Work out the finished part from the listing and answer in its coordinate system (mm). Face numbers are marked on the shaded views. A direction names the side the tool comes from. Round coordinates to 2 decimals unless told otherwise and drop trailing zeros. Order: outer loops, then holes, each group sorted by start corner. A loop starts at its lowest first (then second) coordinate and runs counter-clockwise, first axis right, second up. Notation, with made-up numbers: (60, 88.25) - (97, 88.25) arc R32 ccw to (97, 121.25) - close; hole circle Ø7 at (11.5, -11.75). An arc over 180 degrees is marked (long way). Put each result on its own line as item: value.
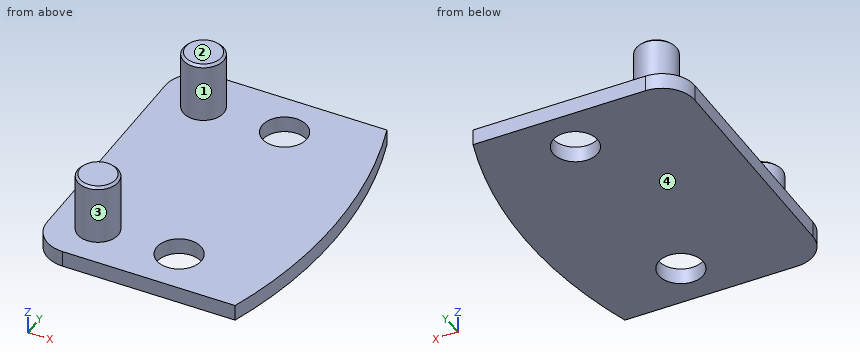
Autodesk Inventor part; units mm, degrees
ref_plane "YZ Plane" through (0, 0, 0) normal (1, 0, 0) x (0, 1, 0)
ref_plane "XZ Plane" through (0, 0, 0) normal (0, 1, 0) x (-1, 0, 0)
ref_plane "XY Plane" through (0, 0, 0) normal (0, 0, 1) x (1, 0, 0)
sketch "Esquisse1" plane through (0, 0, 0) normal (0, 0, 1) x (1, 0, 0)
  line L0 (0, 0) -> (-29, 0)
  line L1 (-29, 0) -> (-29, 36)
  line L2 (-29, 36) -> (0, 36)
  line L3 (-24.5656, 33) -> (-19.5656, 33)
  line L4 (-19.5656, 33) -> (-19.5656, 28)
  line L5 (-19.5656, 28) -> (-24.5656, 28)
  line L6 (-24.5656, 28) -> (-24.5656, 33)
  line L7 (-14.5656, 33) -> (-9.5656, 33)
  line L8 (-9.5656, 33) -> (-9.5656, 28)
  line L9 (-9.5656, 28) -> (-14.5656, 28)
  line L10 (-14.5656, 28) -> (-14.5656, 33)
  line L11 (-24.5656, 8) -> (-19.5656, 8)
  line L12 (-19.5656, 8) -> (-19.5656, 3)
  line L13 (-19.5656, 3) -> (-24.5656, 3)
  line L14 (-24.5656, 3) -> (-24.5656, 8)
  line L15 (-14.5656, 8) -> (-9.5656, 8)
  line L16 (-9.5656, 8) -> (-9.5656, 3)
  line L17 (-9.5656, 3) -> (-14.5656, 3)
  line L18 (-14.5656, 3) -> (-14.5656, 8)
  arc A0 (0, 0) -> (0, 36) centre (-54.0833, 18) ccw
  line L19 (-9.3156, 33.25) -> (-14.8156, 33.25)
  line L20 (-14.8156, 33.25) -> (-14.8156, 27.75)
  line L21 (-14.8156, 27.75) -> (-9.3156, 27.75)
  line L22 (-9.3156, 27.75) -> (-9.3156, 33.25)
  line L23 (-9.3156, 8.25) -> (-14.8156, 8.25)
  line L24 (-14.8156, 8.25) -> (-14.8156, 2.75)
  line L25 (-14.8156, 2.75) -> (-9.3156, 2.75)
  line L26 (-9.3156, 2.75) -> (-9.3156, 8.25)
  dimension "d0" = 36
  dimension "d1" = 29
  dimension "d2" = 5
  dimension "d3" = 5
  dimension "d4" = 5
  dimension "d5" = 5
  dimension "d6" = 20
  dimension "d7" = 5
  dimension "d8" = 3
  dimension "d9" = 57
  dimension "d21" = 5.5
  dimension "d22" = 5.5
extrude "Extrusion1" add sketch "Esquisse1" along normal blind 2 contours L0 L1 L2 A0 | L22 L21 L20 L19 | L26 L25 L24 L23
extrude "Extrusion3" add sketch "Esquisse1" along normal blind 9.5 contours L3 L4 L5 L6 | L11 L12 L13 L14
fillet "Congé1" radius 4 2 edges at (-29, 0, 1) (-29, 36, 1)
sketch "Esquisse2" plane through (0, 0, 2) normal (0, 0, 1) x (1, 0, 0)
  line L0 (-9.5656, 8) -> (-9.5656, 3)
  line L1 (-9.5656, 3) -> (-14.5656, 3)
  line L2 (-14.5656, 3) -> (-14.5656, 8)
  line L3 (-14.5656, 8) -> (-9.5656, 8)
  line L4 (-19.5656, 8) -> (-19.5656, 3)
  line L5 (-19.5656, 3) -> (-24.5656, 3)
  line L6 (-24.5656, 3) -> (-24.5656, 8)
  line L7 (-24.5656, 8) -> (-19.5656, 8)
  line L8 (-9.5656, 33) -> (-9.5656, 28)
  line L9 (-9.5656, 28) -> (-14.5656, 28)
  line L10 (-14.5656, 28) -> (-14.5656, 33)
  line L11 (-14.5656, 33) -> (-9.5656, 33)
  line L12 (-19.5656, 33) -> (-19.5656, 28)
  line L13 (-19.5656, 28) -> (-24.5656, 28)
  line L14 (-24.5656, 28) -> (-24.5656, 33)
  line L15 (-24.5656, 33) -> (-19.5656, 33)
  arc A0 (-25, 36) -> (-29, 32) centre (-25, 32) ccw
  line L16 (-29, 32) -> (-29, 4)
  arc A1 (-29, 4) -> (-25, 0) centre (-25, 4) ccw
  line L17 (-25, 0) -> (0, 0)
  arc A2 (0, 0) -> (0, 36) centre (-54.0833, 18) ccw
  line L18 (0, 36) -> (-25, 36)
  circle A3 centre (-12.0656, 30.5) radius 2.5
  circle A4 centre (-12.0656, 5.5) radius 2.5
extrude "Extrusion4" add sketch "Esquisse2" against normal up to surface (2 mm away) contours L0 A4 L3 | L0 L1 A4 | A4 L2 L3 | L1 L2 A4 | L8 A3 L11 | L8 L9 A3 | A3 L10 L11 | L9 L10 A3
sketch "Esquisse3" plane through (0, 0, 9.5) normal (0, 0, 1) x (1, 0, 0)
  circle A0 centre (-12.0656, 5.5) radius 2.5
  line L0 (-19.5656, 8) -> (-19.5656, 3)
  line L1 (-19.5656, 3) -> (-24.5656, 3)
  line L2 (-24.5656, 3) -> (-24.5656, 8)
  line L3 (-24.5656, 8) -> (-19.5656, 8)
  circle A1 centre (-12.0656, 30.5) radius 2.5
  line L4 (-19.5656, 33) -> (-19.5656, 28)
  line L5 (-19.5656, 28) -> (-24.5656, 28)
  line L6 (-24.5656, 28) -> (-24.5656, 33)
  line L7 (-24.5656, 33) -> (-19.5656, 33)
  arc A2 (-25, 36) -> (-29, 32) centre (-25, 32) ccw
  line L8 (-29, 32) -> (-29, 4)
  arc A3 (-29, 4) -> (-25, 0) centre (-25, 4) ccw
  line L9 (-25, 0) -> (0, 0)
  arc A4 (0, 0) -> (0, 36) centre (-54.0833, 18) ccw
  line L10 (0, 36) -> (-25, 36)
  circle A5 centre (-22.0656, 30.5) radius 2.5
  circle A6 centre (-22.0656, 5.5) radius 2.5
extrude "Extrusion5" cut sketch "Esquisse3" against normal up to surface (7.5 mm away) contours L0 A6 L3 | L0 L1 A6 | A6 L2 L3 | L1 L2 A6 | L4 A5 L7 | L4 L5 A5 | A5 L6 L7 | L5 L6 A5
sketch "Esquisse4" plane through (0, 0, 2) normal (0, 0, 1) x (1, 0, 0)
  circle A0 centre (-12.0656, 5.5) radius 2.5
  circle A1 centre (-22.0656, 5.5) radius 2.5
  circle A2 centre (-12.0656, 30.5) radius 2.5
  circle A3 centre (-22.0656, 30.5) radius 2.5
  arc A4 (-25, 36) -> (-29, 32) centre (-25, 32) ccw
  line L0 (-29, 32) -> (-29, 4)
  arc A5 (-29, 4) -> (-25, 0) centre (-25, 4) ccw
  line L1 (-25, 0) -> (0, 0)
  arc A6 (0, 0) -> (0, 36) centre (-54.0833, 18) ccw
  line L2 (0, 36) -> (-25, 36)
  circle A7 centre (-12.0656, 30.5) radius 2.75
  circle A8 centre (-12.0656, 5.5) radius 2.75
  dimension "d23" = 5.5
  dimension "d24" = 5.5
extrude "Extrusion6" cut sketch "Esquisse4" against normal through all contours A7 | A8
chamfer "Chanfrein1" distance 0.3 angle 45 2 edges at (-24.5656, 5.5, 9.5) (-24.5656, 30.5, 9.5)
sketch "Esquisse5" plane through (0, 0, 0) normal (0, 0, -1) x (-1, 0, 0)
  circle A0 centre (34.0656, -7) radius 1.15
  circle A1 centre (40.5656, -7) radius 1.15
  circle A2 centre (70.5656, -7) radius 1.15
  circle A3 centre (77.0656, -7) radius 1.15
  circle A4 centre (45.5656, 14.75) radius 1.15
  circle A5 centre (65.5656, 14.75) radius 1.15
  circle A6 centre (65.5656, 21.25) radius 1.15
  circle A7 centre (45.5656, 21.25) radius 1.15
  circle A8 centre (77.0656, 43) radius 1.15
  circle A9 centre (70.5656, 43) radius 1.15
  circle A10 centre (40.5656, 43) radius 1.15
  circle A11 centre (34.0656, 43) radius 1.15
  line L0 (40.3656, 10.5) -> (40.3656, 0.5)
  line L1 (70.7477, 10.5) -> (40.3656, 10.5)
  line L2 (70.7477, 0.5) -> (70.7477, 10.5)
  line L3 (66.7656, 0.5) -> (70.7477, 0.5)
  line L4 (66.7656, 0.5) -> (66.7656, -12)
  line L5 (66.7656, -12) -> (82.5656, -12)
  arc A12 (82.5656, -12) -> (86.5656, -8) centre (82.5656, -8) ccw
  line L6 (86.5656, -8) -> (86.5656, 0)
  line L7 (86.5656, 0) -> (87.5656, 0)
  arc A13 (83.5656, 4) -> (87.5656, 0) centre (87.5656, 4) ccw
  line L8 (83.5656, 4) -> (83.5656, 9)
  arc A14 (87.5656, 13) -> (83.5656, 9) centre (87.5656, 9) ccw
  line L9 (87.5656, 13) -> (104.0656, 13)
  arc A15 (105.2725, 12.5947) -> (104.0656, 13) centre (104.0656, 11) ccw
  arc A16 (105.2725, 12.5947) -> (105.2725, 23.4053) centre (55.5656, 18) ccw
  arc A17 (104.0656, 23) -> (105.2725, 23.4053) centre (104.0656, 25) ccw
  line L10 (104.0656, 23) -> (87.5656, 23)
  arc A18 (83.5656, 27) -> (87.5656, 23) centre (87.5656, 27) ccw
  line L11 (83.5656, 27) -> (83.5656, 32)
  arc A19 (87.5656, 36) -> (83.5656, 32) centre (87.5656, 32) ccw
  line L12 (87.5656, 36) -> (86.5656, 36)
  line L13 (86.5656, 36) -> (86.5656, 44)
  arc A20 (86.5656, 44) -> (82.5656, 48) centre (82.5656, 44) ccw
  line L14 (82.5656, 48) -> (66.7656, 48)
  line L15 (66.7656, 48) -> (66.7656, 35.5)
  line L16 (70.7477, 35.5) -> (66.7656, 35.5)
  line L17 (70.7477, 25.5) -> (70.7477, 35.5)
  line L18 (40.3656, 25.5) -> (70.7477, 25.5)
  line L19 (40.3656, 35.5) -> (40.3656, 25.5)
  line L20 (44.3656, 35.5) -> (40.3656, 35.5)
  line L21 (44.3656, 35.5) -> (44.3656, 48)
  line L22 (44.3656, 48) -> (28.5656, 48)
  arc A21 (28.5656, 48) -> (24.5656, 44) centre (28.5656, 44) ccw
  line L23 (24.5656, 44) -> (24.5656, 36)
  line L24 (24.5656, 36) -> (23.5656, 36)
  arc A22 (27.5656, 32) -> (23.5656, 36) centre (23.5656, 32) ccw
  line L25 (27.5656, 32) -> (27.5656, 27)
  arc A23 (23.5656, 23) -> (27.5656, 27) centre (23.5656, 27) ccw
  line L26 (23.5656, 23) -> (7.0656, 23)
  arc A24 (5.8586, 23.4053) -> (7.0656, 23) centre (7.0656, 25) ccw
  arc A25 (5.8586, 23.4053) -> (5.8586, 12.5947) centre (55.5656, 18) ccw
  arc A26 (7.0656, 13) -> (5.8586, 12.5947) centre (7.0656, 11) ccw
  line L27 (7.0656, 13) -> (23.5656, 13)
  arc A27 (27.5656, 9) -> (23.5656, 13) centre (23.5656, 9) ccw
  line L28 (27.5656, 9) -> (27.5656, 4)
  arc A28 (23.5656, 0) -> (27.5656, 4) centre (23.5656, 4) ccw
  line L29 (23.5656, 0) -> (24.5656, 0)
  line L30 (24.5656, 0) -> (24.5656, -8)
  arc A29 (24.5656, -8) -> (28.5656, -12) centre (28.5656, -8) ccw
  line L31 (28.5656, -12) -> (44.3656, -12)
  line L32 (44.3656, -12) -> (44.3656, 0.5)
  line L33 (40.3656, 0.5) -> (44.3656, 0.5)
  line L34 (27.5656, 4) -> (27.5656, 32)
  arc A30 (23.5656, 0) -> (27.5656, 4) centre (23.5656, 4) ccw
  arc A31 (27.5656, 32) -> (23.5656, 36) centre (23.5656, 32) ccw
  line L35 (23.5656, 0) -> (2.3, 0)
  line L36 (25, 0) -> (0, 0)
  line L37 (23.5656, 36.0967) -> (2.3, 36)
  line L38 (25, 36) -> (0, 36)
  arc A32 (2.3, 36) -> (2.3, 0) centre (56.3833, 18) ccw
  arc A33 (0, 36) -> (0, 0) centre (54.0833, 18) ccw
  line L39 (29, 4) -> (29, 32)
  arc A34 (25, 0) -> (29, 4) centre (25, 4) ccw
  arc A35 (29, 32) -> (25, 36) centre (25, 32) ccw
  line L40 (0, 0) -> (25, 0)
  dimension "d30" = 2.3
  dimension "d31" = 2.3
  dimension "d32" = 57
  dimension "d33" = 57
extrude "Extrusion7" cut sketch "Esquisse5" against normal through all contours L29 A28 L28 L34 L25 A22 L24 L38 A35 L39 A34 L36 | L36 A33 L38 A32
properties part number "green_part-july21" material "Plastique ABS"
1) For the marked faces 3 and 4, determine the directions among +Z, -Z, +X, -X, +Y, -Y from which every point of the face is accessible in a straight line to the end or side of a thin tool.
Findings below:
face 3: +Z
face 4: -Z, +X, -X, +Y, -Y
2) A cutting plane is placed at D-D on y = 26. Write down the section's boundary in (x, z), then the cut area to 3 significant figures.
Findings below:
outline: (-27.57, 0) - (0.05, 0) - (0.05, 2) - (-27.57, 2) - close
area: 55.2 mm2
3) A cutting plane is placed at A-A on y = 5.5. Write down the section's boundary in (x, z).
Findings below:
outline: (-27.57, 0) - (-14.82, 0) - (-14.82, 2) - (-19.57, 2) - (-19.57, 9.2) - (-19.87, 9.5) - (-24.27, 9.5) - (-24.57, 9.2) - (-24.57, 2) - (-27.57, 2) - close; (-9.32, 0) - (-0.77, 0) - (-0.77, 2) - (-9.32, 2) - close
4) A cutting plane is placed at C-C on x = -3.5. Write down the section's boundary in (y, z).
Findings below:
outline: (0, 0) - (36, 0) - (36, 2) - (0, 2) - close
5) For a pull along Y with two mould halves and no side action, classify the marked faces 1 and 2 as pulls with the +Y half, pulls with the -Y half, needs draft (parallel to the pull), parting line crosses it, or undercut.
Findings below:
face 1: undercut
face 2: needs draft
6) A cutting plane is placed at B-B on z = 7.75. Write down the section's boundary in (x, y), then the cut area to 3 significant figures.
Findings below:
outline: circle Ø5 at (-22.07, 5.5); circle Ø5 at (-22.07, 30.5)
area: 39.3 mm2
7) Straight lines are drawn through the part: L1, parallel to Z at x = -20, y = 22; L2, parallel to Y at x = -23, z = 2.5; L3, parallel to Y at x = -20.5, z = 3.75. For each, find the intervals that lie inside material, in ascending order. Write a range as from..to.
Findings below:
L1: z = 0..2
L2: y = 3.18..7.82, 28.18..32.82
L3: y = 3.55..7.45, 28.55..32.45
8) Given pin 1 Ø1 at (y, z) = (28.5, 4.5) entering from +X; pin 2 Ø5 at (x, y) = (-7, 19.5) entering from +Z; pin 3 Ø5 at (y, z) = (17.5, 5.5) entering from -X, each flat-ended and moving along its own axis, determine where each tip first touches the part or whether it passes through.
Findings below:
pin 1: stops at x = -20.07
pin 2: stops at z = 2
pin 3: passes through
